The listing builds one solid part. Answer for the finished solid, in the listing's coordinates (mm). Coordinates: 2 decimals unless noted, no trailing zeros. Write each loop counter-clockwise with the first axis right and the second up, starting at its lowest first coordinate (ties: lowest second). Pieces come first, ordered by that corner, then holes.
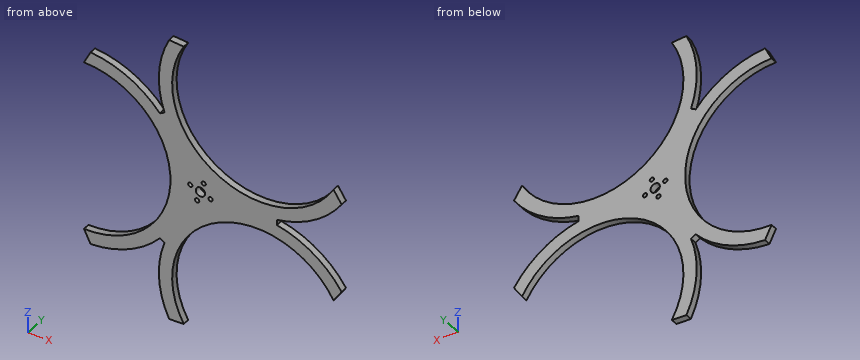
Autodesk Inventor part; units mm, degrees
ref_plane "YZ Plane" through (0, 0, 0) normal (1, 0, 0) x (0, 1, 0)
ref_plane "XZ Plane" through (0, 0, 0) normal (0, 1, 0) x (-1, 0, 0)
ref_plane "XY Plane" through (0, 0, 0) normal (0, 0, 1) x (1, 0, 0)
sketch "Эскиз1" plane through (0, 0, 0) normal (0, 1, 0) x (-1, 0, 0)
  circle A0 centre (0, 0) radius 152.5
  line L0 (0, 0) -> (152.5, 0)
  circle A1 centre (87.5, 0) radius 65
  circle A2 centre (-43.75, 75.7772) radius 65
  circle A3 centre (-43.75, -75.7772) radius 65
  circle A4 centre (87.5, 0) radius 75
  circle A5 centre (-43.75, 75.7772) radius 75
  circle A6 centre (-43.75, -75.7772) radius 75
  line L1 (0, 0) -> (-76.25, 132.0689)
  line L2 (0, 0) -> (-76.25, -132.0689)
  line L3 (144.5, 48.7442) -> (30.5, -48.7442)
  line L4 (-114.4637, 100.7686) -> (26.9637, 50.7859)
  line L5 (-30.0363, -149.5128) -> (-57.4637, -2.0417)
  line L6 (30.5, -48.7442) -> (26.9637, -50.7859)
  line L7 (26.9637, 50.7859) -> (30.5, 48.7442)
  line L8 (-57.4637, -2.0417) -> (-57.4637, 2.0417)
  line L9 (87.5, -75) -> (87.5, 75)
  line L10 (21.2019, 113.2772) -> (-108.7019, 38.2772)
  line L11 (-108.7019, -38.2772) -> (21.2019, -113.2772)
  point P0 (14.0693, 24.3687)
  point P1 (-28.1386, 0)
  point P2 (14.0693, -24.3687)
  point P3 (12.5, 0)
  point P4 (22.5, 0)
  point P5 (152.5, 0)
  point P6 (-6.25, 10.8253)
  point P7 (-11.25, 19.4856)
  point P8 (-76.25, 132.0689)
  point P9 (-114.4637, 100.7686)
  point P10 (-6.25, -10.8253)
  point P11 (-11.25, -19.4856)
  point P12 (-76.25, -132.0689)
  point P13 (-30.0363, -149.5128)
  point P14 (-114.4637, -100.7686)
  point P15 (-30.0363, 149.5128)
  point P16 (144.5, -48.7442)
  point P17 (152.5, 0)
  point P18 (136.9, 42.245)
  point P19 (17.5352, 54.1181)
  point P20 (-105.0352, 97.4364)
  point P21 (-114.4637, 100.7686)
  point P22 (-57.4637, -2.0417)
  point P23 (-55.6352, -11.8731)
  point P24 (-31.8648, -139.6814)
  point P25 (-30.0363, -149.5128)
  point P26 (38.1, -42.245)
  point P27 (87.5, -65)
  point P28 (87.5, 65)
  point P29 (12.5417, 108.2772)
  point P30 (-100.0417, 43.2772)
  point P31 (-57.4637, -2.0417)
  point P32 (-100.0417, -43.2772)
  point P33 (12.5417, -108.2772)
  dimension "d0" = 305
  dimension "d1" = 130
  dimension "d2" = 0
  dimension "d5" = 360
  dimension "d7" = 150
  dimension "d10" = 360
  dimension "d16" = 360
  dimension "d18" = 0
  dimension "d21" = 360
  dimension "d25" = 360
  dimension "d48" = 360
extrude "Выдавливание1" add sketch "Эскиз1" along normal blind 5 contours L9 A4 L3 A1 | L9 A1 L0 A4 | A1 L3 A4 L0 | A5 L4 A2 L10 | A4 L0 L1 A5 L7 | L11 A3 L2 A6 | L6 A6 L2 L0 A4 | L10 A2 L1 A5 | A5 L1 A2 L4 | L11 A6 L5 A3 | L2 A6 L8 A5 L1 | L5 A6 L2 A3 picked at (58.9785, -61.9188) picked at (22.0957, 93.4205) picked at (-83.1125, -20.1174)
sketch "Эскиз4" plane through (0, 5, 0) normal (0, 1, 0) x (1, 0, 0)
  circle A0 centre (0, 0) radius 3.5
  dimension "d43" = 7
extrude "Выдавливание4" cut sketch "Эскиз4" against normal blind 140
sketch "Эскиз5" plane through (0, 5, 0) normal (0, 1, 0) x (1, 0, 0)
  circle A0 centre (0, 0) radius 3.5
  arc A1 (-87.5, -65) -> (-87.5, 65) centre (-87.5, 0) ccw
  line L0 (-87.5, -65) -> (-87.5, -69)
  line L1 (-87.5, -65) -> (-87.5, -75)
  circle A2 centre (0, 0) radius 111.4327
  circle A3 centre (0, 0) radius 192.7389
  dimension "d51" = 4
extrude "Выдавливание5" cut sketch "Эскиз5" against normal through all contours A3
sketch "Эскиз6" plane through (0, 5, 0) normal (0, 1, 0) x (1, 0, 0)
  line L0 (103.5058, 41.2772) -> (100.0417, 43.2772)
  arc A0 (57.4637, 2.0417) -> (106.0924, 34.0829) centre (43.75, 75.7772) ccw
  line L1 (100.0417, 43.2772) -> (106.0924, 34.0829)
  line L2 (-87.5, 65) -> (-82.5629, 74.8373)
  line L3 (-12.5417, -108.2772) -> (-23.5296, -108.9202)
  line L4 (100.0417, -43.2772) -> (103.5058, -41.2772)
  line L5 (106.0924, -34.0829) -> (100.0417, -43.2772)
  line L6 (-23.5296, 108.9202) -> (-12.5417, 108.2772)
  line L7 (-82.5629, -74.8373) -> (-87.5, -65)
  arc A1 (-12.5417, 108.2772) -> (100.0417, 43.2772) centre (43.75, 75.7772) ccw
  arc A2 (-82.5629, 74.8373) -> (-87.5, 69) centre (0, 0) ccw
  line L8 (-87.5, 69) -> (-87.5, 65)
  arc A3 (-87.5, -65) -> (-87.5, 65) centre (-87.5, 0) ccw
  line L9 (-87.5, -65) -> (-87.5, -69)
  arc A4 (-87.5, -69) -> (-82.5629, -74.8373) centre (0, 0) ccw
  arc A5 (-82.5629, -74.8373) -> (-30.5, -48.7442) centre (-87.5, 0) ccw
  line L10 (-30.5, -48.7442) -> (-26.9637, -50.7859)
  arc A6 (-26.9637, -50.7859) -> (-23.5296, -108.9202) centre (43.75, -75.7772) ccw
  arc A7 (-23.5296, -108.9202) -> (-16.0058, -110.2772) centre (0, 0) ccw
  line L11 (-16.0058, -110.2772) -> (-12.5417, -108.2772)
  arc A8 (100.0417, -43.2772) -> (-12.5417, -108.2772) centre (43.75, -75.7772) ccw
  line L12 (100.0417, -43.2772) -> (103.5058, -41.2772)
  arc A9 (103.5058, -41.2772) -> (106.0924, -34.0829) centre (0, 0) ccw
  arc A10 (106.0924, -34.0829) -> (57.4637, -2.0417) centre (43.75, -75.7772) ccw
  line L13 (57.4637, -2.0417) -> (57.4637, 2.0417)
  arc A11 (57.4637, 2.0417) -> (106.0924, 34.0829) centre (43.75, 75.7772) ccw
  arc A12 (106.0924, 34.0829) -> (103.5058, 41.2772) centre (0, 0) ccw
  line L14 (103.5058, 41.2772) -> (100.0417, 43.2772)
  arc A13 (-12.5417, 108.2772) -> (100.0417, 43.2772) centre (43.75, 75.7772) ccw
  line L15 (-12.5417, 108.2772) -> (-16.0058, 110.2772)
  arc A14 (-16.0058, 110.2772) -> (-23.5296, 108.9202) centre (0, 0) ccw
  arc A15 (-23.5296, 108.9202) -> (-26.9637, 50.7859) centre (43.75, 75.7772) ccw
  line L16 (-26.9637, 50.7859) -> (-30.5, 48.7442)
  arc A16 (-30.5, 48.7442) -> (-82.5629, 74.8373) centre (-87.5, 0) ccw
  circle A17 centre (0, 0) radius 3.5
  point P0 (-12.5417, 108.2772)
  point P1 (106.0924, 34.0829)
  dimension "d56" = 360
  dimension "d60" = 360
extrude "Выдавливание6" cut sketch "Эскиз6" against normal through all contours A12 L1 L0 | L6 A14 L15 | A9 L4 L5 | L2 L8 A2 | L11 A7 L3 | L7 A4 L9
sketch "Эскиз7" plane through (0, 5, 0) normal (0, 1, 0) x (1, 0, 0)
  circle A0 centre (7.6092, 2.4699) radius 1.6
  circle A1 centre (-7.6092, -2.4699) radius 1.6
  circle A2 centre (-2.4699, 7.6092) radius 1.6
  circle A3 centre (0, 0) radius 3.1
  circle A4 centre (2.4699, -7.6092) radius 1.6
extrude "Выдавливание7" cut sketch "Эскиз7" against normal through all contours A0 | A1 | A2 | A4
sketch "Эскиз8" plane through (0, 5, 0) normal (0, 1, 0) x (1, 0, 0)
  circle A0 centre (-2.4699, 7.6092) radius 1.6
  circle A1 centre (7.6092, 2.4699) radius 1.6
  circle A2 centre (-7.6092, -2.4699) radius 1.6
  circle A3 centre (2.4699, -7.6092) radius 1.6
  line L0 (-23.5296, -108.9202) -> (-12.5417, -108.2772)
  arc A4 (100.0417, -43.2772) -> (-12.5417, -108.2772) centre (43.75, -75.7772) ccw
  line L1 (100.0417, -43.2772) -> (106.0924, -34.0829)
  arc A5 (106.0924, -34.0829) -> (57.4637, -2.0417) centre (43.75, -75.7772) ccw
  line L2 (57.4637, -2.0417) -> (57.4637, 2.0417)
  arc A6 (57.4637, 2.0417) -> (106.0924, 34.0829) centre (43.75, 75.7772) ccw
  line L3 (106.0924, 34.0829) -> (100.0417, 43.2772)
  arc A7 (-12.5417, 108.2772) -> (100.0417, 43.2772) centre (43.75, 75.7772) ccw
  line L4 (-12.5417, 108.2772) -> (-23.5296, 108.9202)
  arc A8 (-23.5296, 108.9202) -> (-26.9637, 50.7859) centre (43.75, 75.7772) ccw
  line L5 (-26.9637, 50.7859) -> (-30.5, 48.7442)
  arc A9 (-30.5, 48.7442) -> (-82.5629, 74.8373) centre (-87.5, 0) ccw
  line L6 (-82.5629, 74.8373) -> (-87.5, 65)
  arc A10 (-87.5, -65) -> (-87.5, 65) centre (-87.5, 0) ccw
  line L7 (-87.5, -65) -> (-82.5629, -74.8373)
  arc A11 (-82.5629, -74.8373) -> (-30.5, -48.7442) centre (-87.5, 0) ccw
  line L8 (-30.5, -48.7442) -> (-26.9637, -50.7859)
  arc A12 (-26.9637, -50.7859) -> (-23.5296, -108.9202) centre (43.75, -75.7772) ccw
  circle A13 centre (0, 0) radius 3.5
properties part number "сюрикен 2 dthcbz"
1. Section D-D on x = 51.5 is taken. Give the vertices of the cut face in (y, z).
Results found:
outline: (0, -11.24) - (5, -11.24) - (5, 11.24) - (0, 11.24) - close
2. Section A-A on x = 71 is taken. Give the vertices of the cut face in (y, z).
Results found:
outline: (0, -16.77) - (5, -16.77) - (5, -5.9) - (0, -5.9) - close; (0, 5.9) - (5, 5.9) - (5, 16.77) - (0, 16.77) - close
3. Section B-B on z = 40.5 is taken. Give the vertices of the cut face in (x, y), then the cut area to 3 significant figures.
Results found:
outline: (-36.66, 0) - (-10.84, 0) - (-10.84, 5) - (-36.66, 5) - close; (98.34, 0) - (101.87, 0) - (101.87, 5) - (98.34, 5) - close
area: 147 mm2
4. Flat-ended cylindrical pins translate along their axes: P1, Ø1.9, axis at x = -2.47, z = -7.61, coming from the -Y side; P2, Ø1.5, axis at x = 36.5, y = 0.5, coming from the +Z side. Find the tip coordinate at first contact, or state that the pin passes through.
Results found:
P1: passes through
P2: stops at z = 11.27
5. Find the intervals of material crossed by L1, parallel to X at y = 0.45, z = 0; L2, parallel to Z at x = -73.5, y = 4; L3, parallel to Z at x = 89, y = 1.05, in increasing order.
Results found:
L1: x = -22.5 to -3.5, 3.5 to 57.46
L2: z = -73.68 to -63.47, 63.47 to 73.68
L3: z = -29.11 to -15.97, 15.97 to 29.11
